```python
from build123d import *

# Parameters (mm, degrees)
SKETCH1_W            = 635.3556
SKETCH1_H            = 165.1
BOSS_EXTRUDE1_DEPTH  = 1.5875
SKETCH2_W            = 254
SKETCH2_H            = 3.175
BOSS_EXTRUDE2_DEPTH  = 3.175
BOSS_EXTRUDE3_DEPTH  = 3.175
SKETCH5_W            = 1.143
SKETCH5_H            = 107.442
SKETCH5_W_2          = 3.175
SKETCH5_H_2          = 76.2
CUT_EXTRUDE2_DEPTH   = 361.921161502
M6_CLEARANCE_HOLE1_D = 6.6
LPATTERN2_COUNT      = 4
LPATTERN2_PITCH      = 177.8


with BuildPart() as part:
    # Sketch1 → Boss-Extrude1 (new, symmetric)
    with BuildSketch(Plane(origin=(0, 0, 0), x_dir=(1, 0, 0), z_dir=(0, 1, 0))):
        Rectangle(SKETCH1_W, SKETCH1_H)
    extrude(amount=BOSS_EXTRUDE1_DEPTH, both=True)

    # Sketch2 → Boss-Extrude2 (add)
    with BuildSketch(Plane(origin=(0, 0, -82.55), x_dir=(-1, 0, 0), z_dir=(0, 0, -1))):
        with Locations((-157.8229, 0)):
            Rectangle(SKETCH2_W, SKETCH2_H)
        with Locations((157.8229, 0)):
            Rectangle(SKETCH2_W, SKETCH2_H)
    extrude(amount=BOSS_EXTRUDE2_DEPTH)

    # Sketch3 → Boss-Extrude3 (add)
    with BuildSketch(Plane.XZ.offset(1.5875)):
        Polygon((317.6778, -82.55), (350.57842, -82.55), (350.57842, -79.375), (317.6778, -34.925), align=None)
    boss_extrude3 = extrude(amount=-BOSS_EXTRUDE3_DEPTH)

    # Mirror1: Boss-Extrude3 across plane
    add(boss_extrude3.mirror(Plane(origin=(0, 0, 0), x_dir=(0, 0, 1), z_dir=(1, 0, 0))))

    # Sketch5 → Cut-Extrude2 (cut, through all)
    with BuildSketch(Plane.XZ.offset(1.5875)):
        with Locations((0.5715, -28.829)):
            Rectangle(SKETCH5_W, SKETCH5_H)
        with Locations((-0.5715, -28.829)):
            Rectangle(SKETCH5_W, SKETCH5_H)
        with Locations((-316.0903, 44.45)):
            Rectangle(SKETCH5_W_2, SKETCH5_H_2)
        with Locations((316.0903, 44.45)):
            Rectangle(SKETCH5_W_2, SKETCH5_H_2)
    extrude(amount=-CUT_EXTRUDE2_DEPTH, mode=Mode.SUBTRACT)

    # M6 Clearance Hole1 (through all)
    with Locations(Plane(origin=(0, 1.5875, 0), x_dir=(1, 0, 0), z_dir=(0, 1, 0))):
        with Locations((266.7, -73.8124)):
            m6_clearance_hole1 = Hole(M6_CLEARANCE_HOLE1_D / 2)

    # LPattern2: M6 Clearance Hole1 ×4
    with Locations(*[(-i * LPATTERN2_PITCH, 0, 0) for i in range(1, LPATTERN2_COUNT)]):
        add(m6_clearance_hole1, mode=Mode.SUBTRACT)


solid = part.part
```
The listing builds one solid part. Answer for the finished solid, in the listing's coordinates (mm). Round coordinates to 2 decimals unless told otherwise and drop trailing zeros. Write each loop counter-clockwise with the first axis right and the second up, starting at its lowest first coordinate (ties: lowest second). Pieces come first, ordered by that corner, then holes. Notation, with made-up numbers: (0, -18) -> (39, -18) arc R35 ccw to (39, 17) -> close; hole circle Ø4 at (68.5, -7.5). An arc over 180 degrees is marked (long way). Use CSV: the item, a comma, the result in double quotes. Start each with the question number.
(1) Section C-C on x = -10 is taken. Give the vertices of the cut face in (y, z), then the cut area to 3 significant figures.
(2) Section D-D on z = -73 is taken. Give the vertices of the cut face in (x, y).
(3) Each of these flat-tipped pins is pushed along its axis until it touches: pin 1 (1 mm diameter, centred on y = -0.5, z = -84.5, fed in from -X); pin 2 (1 mm diameter, centred on y = -0.5, z = 31.5, fed in from -X); pin 3 (1.6 mm diameter, centred on x = 12, y = -0.5, fed in from -Z). Where does it stop, or does it pass through?
(4) Section A-A on z = -6 is taken. Give the vertices of the cut face in (x, y).
(5) Section B-B on y = 0.1 is taken. Give the vertices of the cut face in (x, z) (3 decimals).
(6) Consider L1, parallel to Z at x = 88.9, y = 0.25 (3 decimals); L2, parallel to X at y = -1.1, z = -20; L3, parallel to X at y = 1.2, z = 69.5. Determine where each line is inside the solid, lowest interval first. Write a range as from..to.
(7) The mould has two halves that part along Y. Classify faces 1 (the face through (-334.36, -0.02, -57.46)), 2 (the face through (5, 1.588, 0)), 3 (the face through (5, -1.588, 0)): released by +Y, released by -Y, zero draft, split by the parting line, or undercut.
A:
1,outline,"(-1.59, -82.55) -> (1.59, -82.55) -> (1.59, 82.55) -> (-1.59, 82.55) -> close"
1,area,"524 mm²"
2,outline,"(-345.86, -1.59) -> (-1.14, -1.59) -> (-1.14, 1.59) -> (-345.86, 1.59) -> close; (1.14, -1.59) -> (345.86, -1.59) -> (345.86, 1.59) -> (1.14, 1.59) -> close"
3,pin 1,"stops at x = -284.82"
3,pin 2,"stops at x = -314.5"
3,pin 3,"stops at z = -82.55"
4,outline,"(-317.68, -1.59) -> (-1.14, -1.59) -> (-1.14, 1.59) -> (-317.68, 1.59) -> close; (1.14, -1.59) -> (317.68, -1.59) -> (317.68, 1.59) -> (1.14, 1.59) -> close"
5,outline,"(-350.578, -82.55) -> (-284.823, -82.55) -> (-284.823, -85.725) -> (-30.823, -85.725) -> (-30.823, -82.55) -> (-1.143, -82.55) -> (-1.143, 24.892) -> (1.143, 24.892) -> (1.143, -82.55) -> (30.823, -82.55) -> (30.823, -85.725) -> (284.823, -85.725) -> (284.823, -82.55) -> (350.578, -82.55) -> (350.578, -79.375) -> (317.678, -34.925) -> (317.678, 6.35) -> (314.503, 6.35) -> (314.503, 82.55) -> (-314.503, 82.55) -> (-314.503, 6.35) -> (-317.678, 6.35) -> (-317.678, -34.925) -> (-350.578, -79.375) -> close; hole circle Ø6.6 at (-266.7, 73.812); hole circle Ø6.6 at (-88.9, 73.812); hole circle Ø6.6 at (88.9, 73.812); hole circle Ø6.6 at (266.7, 73.812)"
6,L1,"z = -85.725..70.512, 77.112..82.55"
6,L2,"x = -317.68..-1.14, 1.14..317.68"
6,L3,"x = -314.5..314.5"
7,face 1,"zero draft"
7,face 2,"released by +Y"
7,face 3,"released by -Y"
